```python
from build123d import *

# Parameters (mm, degrees)
SKETCH1_R           = 3
BOSS_EXTRUDE1_DEPTH = 3.3
SKETCH2_R           = 1.5
BOSS_EXTRUDE2_DEPTH = 3.6
SKETCH4_R           = 0.5
BOSS_EXTRUDE4_DEPTH = 0.15
SKETCH3_R           = 0.25


with BuildPart() as part:
    # Sketch1 → Boss-Extrude1 (new body)
    with BuildSketch(Plane(origin=(0, 0, 0), x_dir=(1, 0, 0), z_dir=(0, 1, 0))):
        Circle(SKETCH1_R)
    extrude(amount=BOSS_EXTRUDE1_DEPTH)

    # Sketch2 → Boss-Extrude2 (add)
    with BuildSketch(Plane(origin=(0, 3.3, 0), x_dir=(1, 0, 0), z_dir=(0, 1, 0))):
        Circle(SKETCH2_R)
    extrude(amount=BOSS_EXTRUDE2_DEPTH)

    # Sketch4 → Boss-Extrude4 (add)
    with BuildSketch(Plane(origin=(0, 3.3, 0), x_dir=(1, 0, 0), z_dir=(0, 1, 0))):
        with Locations((-1.60267659, 1.60267659)):
            Circle(SKETCH4_R)
        with Locations((1.60267659, 1.60267659)):
            Circle(SKETCH4_R)
        with Locations((-1.60267659, -1.60267659)):
            Circle(SKETCH4_R)
        with Locations((1.60267659, -1.60267659)):
            Circle(SKETCH4_R)
    extrude(amount=BOSS_EXTRUDE4_DEPTH)

    # Sweep2: sweep along a path in Sketch5
    with BuildLine(Plane.XY) as sweep2_path:
        Line((0, 0), (0, -0.442064994))
        ThreePointArc((0, -0.442064994), (0.152240935, -1.207431859), (0.585786438, -1.856278556))
        Line((0.585786438, -1.856278556), (3.261520237, -4.532012355))
    # Sketch3 → Sweep2 (sweep)
    with BuildSketch(Plane.XZ):
        with Locations((0, 2.6)):
            Circle(SKETCH3_R)
        with Locations((0, -2.6)):
            Circle(SKETCH3_R)
    sweep(path=sweep2_path.line)


solid = part.part
```
Design review of the part built by this model. Coordinates are the model's own, in mm. A direction names the side the tool comes from. Give positions to 0.01 mm unless a question says otherwise; leave off trailing zeros. Write each loop counter-clockwise with the first axis right and the second up, starting at its lowest first coordinate (ties: lowest second). Pieces come first, ordered by that corner, then holes. Notation, with made-up numbers: (-12, -16.5) -> (46, -16.5) arc R19 ccw to (46, 13.5) -> close; hole circle Ø4 at (-11.5, 55.25). An arc over 180 degrees is marked (long way). Answer in a Markdown table with one row per item.
(1) Consider section C-C (x = 1.25). Count the separate pieces of the cut face and the enclosed holes in it, then the cut area to 3 significant figures.
Results:
| item | result |
|---|---|
| separate pieces | 3 |
| enclosed holes | 0 |
| area | 24.7 mm2 |
(2) Mouldability with a two-part tool opening along Z and no side actions: class faces 4 (the cylindrical face through (-3, 2, 0)), 5 (the flat face through (-1.6, 3.45, 1.6)), 6 (the cylindrical face through (1.904, -3.251, -2.844)), 7 (the cylindrical face through (1.81, -3.34, 2.77)) as +Z half, -Z half, draft (parallel to the pull), parting line (faces both ways), or undercut.
Results:
| item | result |
|---|---|
| face 4 | parting line |
| face 5 | draft |
| face 6 | undercut |
| face 7 | undercut |
(3) Consider section D-D (y = 5.25). State the section outline as (x, z) points.
Results:
| item | result |
|---|---|
| outline | circle Ø3 at (0, 0) |
(4) Consider section A-A (z = 0). State the section outline as (x, y) points, then the cut area to 3 significant figures.
Results:
| item | result |
|---|---|
| outline | (-3, 0) -> (3, 0) -> (3, 3.3) -> (1.5, 3.3) -> (1.5, 6.9) -> (-1.5, 6.9) -> (-1.5, 3.3) -> (-3, 3.3) -> close |
| area | 30.6 mm2 |
(5) For faces 1 (the cylindrical face through (-1.5, 5.07, -0.07)), 2 (the flat face through (1.6, 3.45, -1.6)), 3 (the flat face through (1.6, 3.45, 1.6)), list the 3-axis set-ups (+Z, -Z, +X, -X, +Y, -Y) from which the entire face can be reached by the end or side of a thin tool; tool diameter is ignored.
Results:
| item | result |
|---|---|
| face 1 | +Y |
| face 2 | -Z, +X, +Y |
| face 3 | +Z, +X, +Y |
(6) Clearance check with flat-ended pins moving along their axes: pin 1 (1.5 mm diameter, centred on y = 5, z = -1, fed in from -X); pin 2 (1 mm diameter, centred on x = 1.5, z = -1.5, fed in from +Y); pin 3 (2 mm diameter, centred on x = 2, z = -1, fed in from -Y). State where each tip first meets the part, or that it passes through.
Results:
| item | result |
|---|---|
| pin 1 | x = -1.48 |
| pin 2 | y = 3.45 |
| pin 3 | y = 0 |
(7) To check wall thickness, follow probe 1 along Y at (x, z) = (0, -2.2); probe 2 along Z at (x, y) = (0, 5); probe 3 along Y at (x, z) = (0.5, -2.5). State the ranges of each line that lie inside material, in increasing order.
Results:
| item | result |
|---|---|
| probe 1 | 0 to 3.3 |
| probe 2 | -1.5 to 1.5 |
| probe 3 | -2.09 to -1.38, 0 to 3.3 |
(8) Consider section B-B (x = -1.75). State the section outline as (y, z) points.
Results:
| item | result |
|---|---|
| outline | (0, -2.44) -> (3.3, -2.44) -> (3.3, -2.08) -> (3.45, -2.08) -> (3.45, -1.12) -> (3.3, -1.12) -> (3.3, 1.12) -> (3.45, 1.12) -> (3.45, 2.08) -> (3.3, 2.08) -> (3.3, 2.44) -> (0, 2.44) -> close |
